from build123d import *

# Parameters (mm, degrees)
SKETCH_2_W          = 30
SKETCH_2_H          = 23
EXTRUDE_1_DEPTH     = 12
CUT_EXTRUDE_1_DEPTH = 6
SKETCH_4_W          = 15.467270909
SKETCH_4_H          = 13.987209034
CUT_EXTRUDE_2_DEPTH = 40.66106403
SKETCH_5_R          = 1.5
CUT_EXTRUDE_3_DEPTH = 8
SKETCH_6_R          = 1.5
CUT_EXTRUDE_4_DEPTH = 12


with BuildPart() as part:
    # 草图2 → 凸台-拉伸1 (new body)
    with BuildSketch(Plane.XY):
        with Locations((15, 11.5)):
            Rectangle(SKETCH_2_W, SKETCH_2_H)
    extrude(amount=EXTRUDE_1_DEPTH)

    # 草图3 → 切除-拉伸1 (cut)
    with BuildSketch(Plane.XY.offset(12)):
        Polygon((-0.106519248, 5.265031781), (32.137743655, 5.265031781), (32.137743655, 3.165031781), (26.814729775, 3.165031781), (25.621504988, -0.36450698), (22.621504988, -0.36450698), (21.382763952, 3.273233944), (17.391329844, 3.265031781), (16.891449339, 4.265031781), (16.391449339, 4.265031781), (15.891568834, 3.265031781), (15.391568834, 3.265031781), (14.891688328, 4.265031781), (14.391688328, 4.265031781), (13.891807823, 3.265031781), (13.391807823, 3.265031781), (12.891927318, 4.265031781), (12.391927318, 4.265031781), (11.892046813, 3.265031781), (11.392046813, 3.265031781), (10.892166308, 4.265031781), (10.392166308, 4.265031781), (9.892285803, 3.265031781), (9.392285803, 3.265031781), (8.892405298, 4.265031781), (8.392405298, 4.265031781), (7.892524793, 3.265031781), (7.392524793, 3.265031781), (6.892644288, 4.265031781), (6.392644288, 4.265031781), (5.892763783, 3.265031781), (5.392763783, 3.265031781), (4.892883278, 4.265031781), (4.392883278, 4.265031781), (3.893002773, 3.265031781), (3.393002773, 3.265031781), (2.893122268, 4.265031781), (2.260638047, 4.265031781), (1.893241763, 3.265031781), (1.393241763, 3.265031781), (0.893361258, 4.265031781), (0.393361258, 4.265031781), (-0.106519248, 3.265031781), align=None)
    extrude(amount=-CUT_EXTRUDE_1_DEPTH, mode=Mode.SUBTRACT)

    # 草图4 → 切除-拉伸2 (cut, through all)
    with BuildSketch(Plane.XY.offset(12)):
        with Locations((27.733635454, 18.258636298)):
            Rectangle(SKETCH_4_W, SKETCH_4_H)
    extrude(amount=-CUT_EXTRUDE_2_DEPTH, mode=Mode.SUBTRACT)

    # 草图5 → 切除-拉伸3 (cut)
    with BuildSketch(Plane(origin=(0, 11.265031781, 0), x_dir=(1, 0, 0), z_dir=(0, 1, 0))):
        with Locations(Location((24.410160755, -9.07584536, 0), (0, 0, 270))):
            Circle(SKETCH_5_R)
    extrude(amount=-CUT_EXTRUDE_3_DEPTH, mode=Mode.SUBTRACT)

    # 草图6 → 切除-拉伸4 (cut)
    with BuildSketch(Plane(origin=(0, 23, 0), x_dir=(1, 0, 0), z_dir=(0, 1, 0))):
        with Locations(Location((4, -6, 0), (0, 0, 270))):
            Circle(SKETCH_6_R)
        with Locations(Location((16, -6, 0), (0, 0, 90))):
            Circle(SKETCH_6_R)
    extrude(amount=-CUT_EXTRUDE_4_DEPTH, mode=Mode.SUBTRACT)


solid = part.part
Geometry check sheet. Reference: the model listing, model coordinates, mm. A direction names the side the tool comes from. Give positions to 0.01 mm unless a question says otherwise; leave off trailing zeros. Loops run counter-clockwise (first coordinate to the right, second up) from the corner with the lowest first, then second, coordinate; pieces in that order, holes last.
(1) Release check for a two-part mould opening along Y. For faces 5 (the flat face through (13.145, 3.758, 9.042)), 6 (the flat face through (10, 23, 6)), 7 (the flat face through (30, 6, 6)) record: released by +Y, released by -Y, zero draft, split by the parting line, or undercut.
From the geometry:
face 5: undercut
face 6: released by +Y
face 7: zero draft
(2) Depth check by flat-ended pin: pin 1 Ø2.5 at (x, z) = (4, 6) entering from +Y; pin 2 Ø5 at (x, z) = (24.41, 9.08) entering from +Y. Enter the tip coordinate at first touch or a pass-through.
From the geometry:
pin 1: stops at y = 11
pin 2: stops at y = 11.27
(3) Section check A-A on y = 11.75. Record the cut outline in (x, z).
From the geometry:
outline: (0, 0) - (20, 0) - (20, 12) - (0, 12) - close; hole circle Ø3 at (4, 6); hole circle Ø3 at (16, 6)
(4) Thickness scan on L1, parallel to X at y = 21, z = 6; L2, parallel to Z at x = 16, y = 15.5; L3, parallel to Y at x = 9.75, z = 11. Record the ranges inside material, lowest first.
From the geometry:
L1: x = 0 to 2.5, 5.5 to 14.5, 17.5 to 20
L2: z = 0 to 4.5, 7.5 to 12
L3: y = 0 to 3.27, 5.27 to 23
(5) Section check D-D on z = 10.25. Count the separate pieces of the cut face and the enclosed holes in it, then the cut area to 3 significant figures.
From the geometry:
separate pieces: 4
enclosed holes: 0
area: 496 mm2
(6) Set-up check for faces 1 (the flat face through (20, 17, 6)), 2 (the flat face through (28, 3.165, 9)), 3 (the flat face through (16, 11, 6)), 4 (the flat face through (2.08, 3.77, 9.04)): record each of +Z, -Z, +X, -X, +Y, -Y from which the full face is reachable in a straight line by a thin tool's end or side.
From the geometry:
face 1: +Z, -Z, +X, +Y
face 2: +Z, +X
face 3: +Y
face 4: +Z
(7) Section check C-C on z = 5. Record the cut outline in (x, y).
From the geometry:
outline: (0, 0) - (30, 0) - (30, 11.27) - (20, 11.27) - (20, 23) - (17.12, 23) - (17.12, 11) - (14.88, 11) - (14.88, 23) - (5.12, 23) - (5.12, 11) - (2.88, 11) - (2.88, 23) - (0, 23) - close
(8) Section check B-B on x = 23.5. Record the cut outline in (y, z).
From the geometry:
outline: (0, 0) - (11.27, 0) - (11.27, 7.88) - (5.27, 7.88) - (5.27, 6) - (0, 6) - close; (5.27, 10.27) - (11.27, 10.27) - (11.27, 12) - (5.27, 12) - close
